Check sheet for the modelled part. Datum: model origin and axes. Units: mm. Face numbers are marked on the shaded views. A direction names the side the tool comes from. Round coordinates to 2 decimals unless told otherwise and drop trailing zeros. Order: outer loops, then holes, each group sorted by start corner. A loop starts at its lowest first (then second) coordinate and runs counter-clockwise, first axis right, second up.
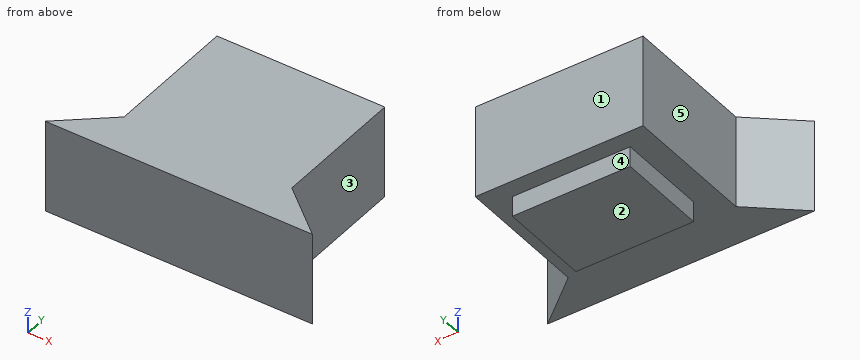
```python
from build123d import *

# Parameters (mm, degrees)
F0_W     = 517.525
F0_H     = 400.05
F1_DEPTH = 88.9
F3_DEPTH = 406.4


with BuildPart() as f1:
    # F0 (on Top) → F1 (new body)
    with BuildSketch(Plane.XY):
        with Locations((258.7625, 176.492612)):
            Rectangle(F0_W, F0_H)
    extrude(amount=F1_DEPTH)

    # F2 (on face) → F3 (join)
    with BuildSketch(Plane.XY.offset(88.9)):
        Polygon((-109.5375, -315.632388), (627.0625, -315.632388), (627.0625, -132.547782), (258.7625, 176.492612), (-109.5375, -132.547782), align=None)
        Polygon((627.0625, -132.547782), (627.0625, -315.632388), (845.254237, -315.632388), align=None)
        Polygon((-327.729237, -315.632388), (-109.5375, -315.632388), (-109.5375, -132.547782), align=None)
        Polygon((258.7625, 176.492612), (627.0625, -132.547782), (627.0625, 452.717612), (-109.5375, 452.717612), (-109.5375, -132.547782), align=None)
    extrude(amount=F3_DEPTH)


solid = f1.part
```
Item 1: Sectioned sample at D-D (z = 69). Record the cut outline in (x, y) (3 decimals), and give its area (3 significant figures).
Answer:
outline: (0, -23.532) - (517.525, -23.532) - (517.525, 376.518) - (0, 376.518) - close
area: 207,000 mm2
Item 2: Sectioned sample at C-C (z = 350.5). Record the cut outline in (x, y), and give its area (3 significant figures).
Answer:
outline: (-327.73, -315.63) - (845.25, -315.63) - (627.06, -132.55) - (627.06, 452.72) - (-109.54, 452.72) - (-109.54, -132.55) - close
area: 606,000 mm2
Item 3: Sectioned sample at B-B (y = 133). Record the cut outline in (x, z) (1 decimal).
Answer:
outline: (-109.5, 88.9) - (0, 88.9) - (0, 0) - (517.5, 0) - (517.5, 88.9) - (627.1, 88.9) - (627.1, 495.3) - (-109.5, 495.3) - close
Item 4: Sectioned sample at A-A (x = 404.5). Record the cut outline in (y, z).
Answer:
outline: (-315.63, 88.9) - (-23.53, 88.9) - (-23.53, 0) - (376.52, 0) - (376.52, 88.9) - (452.72, 88.9) - (452.72, 495.3) - (-315.63, 495.3) - close
Item 5: Go/stop test with flat-tipped pins: P1, Ø8, axis at y = -199.5, z = 373.5, coming from the +X side; P2, Ø1, axis at y = 346.5, z = 235.5, coming from the -X side; P3, Ø12, axis at y = 185.5, z = 85.5, coming from the +X side. Record where each tip stops, or that it passes through.
Answer:
P1: stops at x = 711.62
P2: stops at x = -109.54
P3: stops at x = 627.06
Item 6: Scan lines: line 1 along X through (y, z) = (321, 200); line 2 along Z through (x, y) = (-108, -230); line 3 along Y through (x, z) = (115, 73). Record each from-to range of solid material in increasing order.
Answer:
line 1: x = -109.54 to 627.06
line 2: z = 88.9 to 495.3
line 3: y = -23.53 to 376.52
Item 7: Access from +Z, -Z, +X, -X, +Y, -Y to the whole of each face (thin tool, end or side, straight path). Record for the marked faces 1, 2, 3, 4 and 5.
Answer:
face 1: +Z, -Z, +X, -X, +Y
face 2: -Z, +X, -X, +Y, -Y
face 3: +Z, -Z, +X, +Y
face 4: -Z, +X, -X, +Y
face 5: +Z, -Z, -X, +Y
